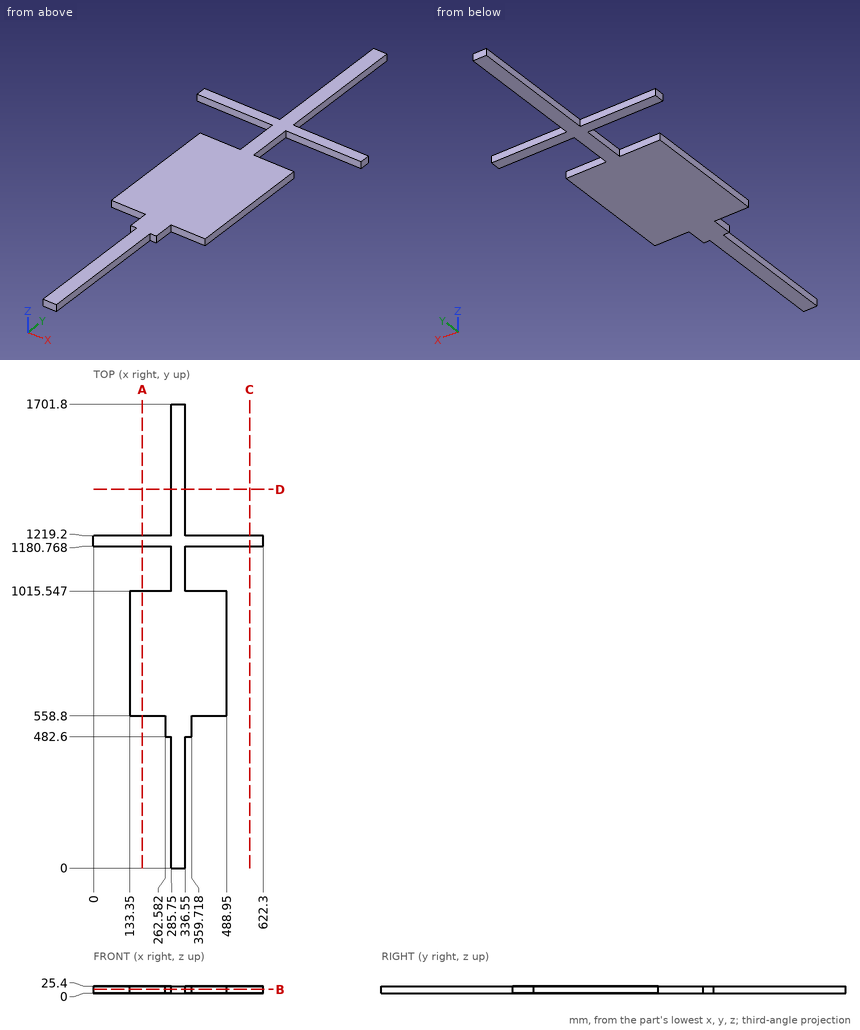
Could you check a few things on this drawing? It's one solid part, dimensions in mm from its lowest x, y, z. Coordinates: 2 decimals unless noted, no trailing zeros. Loops run counter-clockwise (first coordinate to the right, second up) from the corner with the lowest first, then second, coordinate; pieces in that order, holes last.
1. Imagine slicing it at C-C (x = 572.5). Please give me the cut outline in (y, z), and give its area (3 significant figures).
2. Imagine slicing it at A-A (x = 179). Please give me the cut outline in (y, z).
3. For P1, Ø3, axis at x = 105, z = 16.5, coming from the -Y side; P2, Ø12.5, axis at y = 1064.5, z = 13.5, coming from the -X side; P3, Ø12.5, axis at x = 478.5, z = 10, coming from the -Y side; P4, Ø12, axis at x = 452.5, y = 1021, coming from the -Z side, each with a flat end and sliding along its axis, tell me the tip position at first contact or that it passes through.
4. I need wall thicknesses on L1, parallel to Y at x = 364, z = 18; L2, parallel to Y at x = 347, z = 11; L3, parallel to X at y = 1355, z = 14. Which ranges of each line are inside material? Lowest first, please.
5. Imagine slicing it at B-B (z = 13.5). Please give me the cut outline in (x, y), and give its area (3 significant figures).
6. Imagine slicing it at D-D (y = 1388.5). Please give me the cut outline in (x, z).
Computed values:
1. outline: (1180.77, 0) - (1219.2, 0) - (1219.2, 25.4) - (1180.77, 25.4) - close
1. area: 976 mm2
2. outline: (558.8, 0) - (1015.55, 0) - (1015.55, 25.4) - (558.8, 25.4) - close; (1180.77, 0) - (1219.2, 0) - (1219.2, 25.4) - (1180.77, 25.4) - close
3. P1: stops at y = 1180.77
3. P2: stops at x = 285.75
3. P3: stops at y = 558.8
3. P4: stops at z = 0
4. L1: y = 558.8 to 1015.55, 1180.77 to 1219.2
4. L2: y = 482.6 to 1015.55, 1180.77 to 1219.2
4. L3: x = 285.75 to 336.55
5. outline: (0, 1180.77) - (285.75, 1180.77) - (285.75, 1015.55) - (133.35, 1015.55) - (133.35, 558.8) - (262.58, 558.8) - (262.58, 482.6) - (285.75, 482.6) - (285.75, 0) - (336.55, 0) - (336.55, 482.6) - (359.72, 482.6) - (359.72, 558.8) - (488.95, 558.8) - (488.95, 1015.55) - (336.55, 1015.55) - (336.55, 1180.77) - (622.3, 1180.77) - (622.3, 1219.2) - (336.55, 1219.2) - (336.55, 1701.8) - (285.75, 1701.8) - (285.75, 1219.2) - (0, 1219.2) - close
5. area: 251,000 mm2
6. outline: (285.75, 0) - (336.55, 0) - (336.55, 25.4) - (285.75, 25.4) - close
